```python
from build123d import *

# Parameters (mm, degrees)
ESTRUSIONE_ESTRUSIONE3_DEPTH = 30
ESTRUSIONE_ESTRUSIONE4_DEPTH = 25
FORO_18_0_18_1_D             = 18
FORO_10_0_10_1_D             = 10
RACCORDO1_R                  = 5
RACCORDO2_R                  = 2


with BuildPart() as part:
    # Schizzo1 → Estrusione-Estrusione3 (new, symmetric)
    with BuildSketch(Plane.XY):
        with BuildLine():
            ThreePointArc((-1.5, 24.954959427), (-6.644564975, 24.100824805), (-11.5, 22.19797288))
            ThreePointArc((-11.5, 22.19797288), (-24.289394002, -5.918220932), (0, -25))
            ThreePointArc((0, -25), (17.67766953, -17.67766953), (25, 0))
            ThreePointArc((25, 0), (21.360009363, 12.990381057), (11.5, 22.19797288))
            ThreePointArc((11.5, 22.19797288), (6.644564975, 24.100824805), (1.5, 24.954959427))
            Line((1.5, 24.954959427), (1.5, 14.924811557))
            ThreePointArc((1.5, 14.924811557), (11.124297731, 10.062305899), (15, 0))
            ThreePointArc((15, 0), (-10.062305899, -11.124297731), (-1.5, 14.924811557))
            Line((-1.5, 14.924811557), (-1.5, 24.954959427))
        make_face()
    extrude(amount=ESTRUSIONE_ESTRUSIONE3_DEPTH, both=True)

    # Schizzo1_3 → Estrusione-Estrusione4 (add, symmetric)
    with BuildSketch(Plane.XY):
        with BuildLine():
            ThreePointArc((25, 0), (17.67766953, -17.67766953), (0, -25))
            Line((0, -25), (97, -25))
            Line((97, -25), (97, -9.075188443))
            Line((97, -9.075188443), (40, -9.075188443))
            Line((40, -9.075188443), (40, 8.924811557))
            Line((40, 8.924811557), (97, 8.924811557))
            Line((97, 8.924811557), (97, 24.924811557))
            Line((97, 24.924811557), (11.5, 24.924811557))
            Line((11.5, 24.924811557), (11.5, 22.19797288))
            ThreePointArc((11.5, 22.19797288), (21.360009363, 12.990381057), (25, 0))
        make_face()
        with BuildLine():
            Line((1.5, 44.924811557), (1.5, 24.954959427))
            ThreePointArc((1.5, 24.954959427), (6.644564975, 24.100824805), (11.5, 22.19797288))
            Line((11.5, 22.19797288), (11.5, 24.924811557))
            Line((11.5, 24.924811557), (11.5, 44.924811557))
            Line((11.5, 44.924811557), (1.5, 44.924811557))
        make_face()
        with BuildLine():
            Line((-11.5, 44.924811557), (-11.5, 22.19797288))
            ThreePointArc((-11.5, 22.19797288), (-6.644564975, 24.100824805), (-1.5, 24.954959427))
            Line((-1.5, 24.954959427), (-1.5, 44.924811557))
            Line((-1.5, 44.924811557), (-11.5, 44.924811557))
        make_face()
    extrude(amount=ESTRUSIONE_ESTRUSIONE4_DEPTH, both=True)

    # Foro _18.0 _18_-1 (through all)
    with Locations(Plane(origin=(0, -25, 0), x_dir=(-1, 0, 0), z_dir=(0, -1, 0))):
        with Locations((-72, 0)):
            Hole(FORO_18_0_18_1_D / 2)

    # Foro _10.0 _10_-1 (through all)
    with Locations(Plane.ZY.offset(11.5)):
        with Locations((15, 34.924811557), (-15, 34.924811557)):
            Hole(FORO_10_0_10_1_D / 2)

    # Raccordo1
    raccordo1_edges = [part.edges().sort_by_distance(p)[0] for p in [
        (6.5, 44.924811557, -25),
        (6.5, 44.924811557, 25),
        (-6.5, 44.924811557, 25),
        (-6.5, 44.924811557, -25),
    ]]
    fillet(raccordo1_edges, radius=RACCORDO1_R)

    # Raccordo2
    raccordo2_edges = [part.edges().sort_by_distance(p)[0] for p in [
        (40, -9.075188443, -12.5),
        (40, 8.924811557, -12.5),
    ]]
    fillet(raccordo2_edges, radius=RACCORDO2_R)


solid = part.part
```
Can you work these out from the model? Positions are in its coordinate system, mm. A direction names the side the tool comes from. Give positions to 0.01 mm unless a question says otherwise; leave off trailing zeros. Order: outer loops, then holes, each group sorted by start corner. A loop starts at its lowest first (then second) coordinate and runs counter-clockwise, first axis right, second up. Notation, with made-up numbers: M 76,16 L 131,16 A14 cw 131,22 Z; hole C 75.25,0 d9. An arc over 180 degrees is marked long. Write item = value, one per line. Start each with the question number.
Q1. Suppose I cut it at D-D (y = 17). Write out the boundary of the cut face in (x, z), plus the area to 3 significant figures.
Q2. We'd pull the mould along X, two halves only. Please class faces 4 (the flat face through (11.5, 35, 0)), 5 (the flat face through (1.5, 30, 0)), 6 (the flat face through (37, 1, -25)): pulls with the +X half, pulls with the -X half, needs draft (parallel to the pull), parting line crosses it, or undercut.
Q3. I need wall thicknesses on probe 1 along Y at (x, z) = (-9, 15); probe 2 along X at (y, z) = (10, 5.5); probe 3 along Y at (x, z) = (-7, 15). Which ranges of each line are inside material? Lowest first, please. Write a range as [from, to].
Q4. Suppose I cut it at C-C (x = 72). Write out the boundary of the cut face in (y, z).
Q5. For faces 1 (the flat face through (-11.5, 34, 0)), 2 (the cylindrical face through (-6.43, 30.044, 16.084)), 3 (the flat face through (64, -9.075, 6)), which set-ups out of +Z, -Z, +X, -X, +Y, -Y let a thin tool reach every point of the face, with its end or its side?
Q6. Suppose I cut it at B-B (z = 0). Write out the boundary of the cut face in (x, y), plus the area to 3 significant figures.
Q7. Will these pins go through, and if not, where does the flat tip stop? pin 1 Ø13 at (y, z) = (34.92, -15) entering from -X; pin 2 Ø8 at (x, y) = (-4.5, 32.5) entering from -Z; pin 3 Ø15 at (x, z) = (58, 10.5) entering from +Y.
Q8. Suppose I cut it at A-A (y = 28). Write out the boundary of the cut face in (x, z), plus the area to 3 significant figures.
Check result:
q1.outline = M -18.33,-30 L -1.5,-30 L -1.5,30 L -18.33,30 Z; M 1.5,-30 L 18.33,-30 L 18.33,-25 L 97,-25 L 97,25 L 18.33,25 L 18.33,30 L 1.5,30 Z; hole C 72,0 d18
q1.area = 5,700 mm2
q2.face_4 = pulls with the +X half
q2.face_5 = undercut
q2.face_6 = needs draft
q3.probe_1 = [-23.32, -12], [12, 29.92], [39.92, 44.92]
q3.probe_2 = [-22.91, -11.18], [11.18, 64.88], [79.12, 97]
q3.probe_3 = [-24, -13.27], [13.27, 29.92], [39.92, 44.92]
q4.outline = M -25,-25 L -9.08,-25 L -9.08,-9 L -25,-9 Z; M -25,9 L -9.08,9 L -9.08,25 L -25,25 Z; M 8.92,-25 L 24.92,-25 L 24.92,-9 L 8.92,-9 Z; M 8.92,9 L 24.92,9 L 24.92,25 L 8.92,25 Z
q5.face_1 = +Z, -Z, -X, +Y
q5.face_2 = +X, -X
q5.face_3 = +Z, -Z, +X
q6.outline = M -11.5,22.2 A25 ccw 0,-25 L 63,-25 L 63,-9.08 L 42,-9.08 A2 cw 40,-7.08 L 40,6.92 A2 cw 42,8.92 L 63,8.92 L 63,24.92 L 11.5,24.92 L 11.5,44.92 L 1.5,44.92 L 1.5,14.92 A15 cw long -1.5,14.92 L -1.5,44.92 L -11.5,44.92 Z; M 81,-25 L 97,-25 L 97,-9.08 L 81,-9.08 Z; M 81,8.92 L 97,8.92 L 97,24.92 L 81,24.92 Z
q6.area = 3,900 mm2
q7.pin_1 = -11.5
q7.pin_2 = -25
q7.pin_3 = 24.92
q8.outline = M -11.5,-25 L -1.5,-25 L -1.5,25 L -11.5,25 Z; M 1.5,-25 L 11.5,-25 L 11.5,25 L 1.5,25 Z
q8.area = 1,000 mm2
